Check sheet for the modelled part. Datum: model origin and axes. Units: mm. Face numbers are marked on the shaded views. Round coordinates to 2 decimals unless told otherwise and drop trailing zeros. Write each loop counter-clockwise with the first axis right and the second up, starting at its lowest first coordinate (ties: lowest second). Pieces come first, ordered by that corner, then holes. Notation, with made-up numbers: (9, 0) -> (13, 0) arc R22 ccw to (13, 32) -> close; hole circle Ø6 at (-16.5, -37). An arc over 180 degrees is marked (long way). Answer as a JSON object with one key per item and string values. Group by question number.
```python
from build123d import *

# Parameters (mm, degrees)
SKETCH_1_W               = 45
SKETCH_1_H               = 45
EXTRUDE_1_DEPTH          = 4
SKETCH_2_R               = 7.5
CUT_EXTRUDE_1_DEPTH      = 33.070235422
CUT_EXTRUDE_START        = -4.5
SKETCH_4_R               = 1.1
CUT_EXTRUDE_3_DEPTH      = 51.888424881
SKETCH_10_R              = 0.4
CUT_EXTRUDE_9_DEPTH      = 2
SKETCH_7_R               = 1.1
CUT_EXTRUDE_5_DEPTH      = 52.18645266
SKETCH_11_R              = 0.4
CUT_EXTRUDE_10_DEPTH     = 2
CUT_EXTRUDE_4_DEPTH      = 2
PATTERN_CIRCULAR_1_COUNT = 2
SKETCH_6_R               = 1.5
CUT_EXTRUDE_6_DEPTH      = 33.070235434
SKETCH_8_R               = 4.25
CUT_EXTRUDE_7_DEPTH      = 33.070235434
SKETCH_9_R               = 6
CUT_EXTRUDE_8_DEPTH      = 1
SKETCH_12_R              = 1.4
CUT_EXTRUDE_11_DEPTH     = 33.070235434
CHAMFER_1_SIZE           = 1
CHAMFER_2_SIZE           = 1
CHAMFER_3_SIZE           = 2


with BuildPart() as part:
    # 草图1 → 凸台-拉伸1 (new body)
    with BuildSketch(Plane(origin=(0, 0, 0), x_dir=(1, 0, 0), z_dir=(0, 1, 0))):
        Rectangle(SKETCH_1_W, SKETCH_1_H)
    extrude(amount=EXTRUDE_1_DEPTH)

    # 草图2 → 切除-拉伸1 (cut, through all)
    with BuildSketch(Plane(origin=(0, 4, 0), x_dir=(1, 0, 0), z_dir=(0, 1, 0))):
        with Locations(Location((0, 3, 0), (0, 0, 270))):
            Circle(SKETCH_2_R)
    extrude(amount=-CUT_EXTRUDE_1_DEPTH, mode=Mode.SUBTRACT)

    # 草图4 → 切除-拉伸3 (cut)
    with BuildSketch(Plane(origin=(-11.782001231, 4, -8.494037403), x_dir=(-0.4226182617407036, 0, 0.9063077870366482), z_dir=(-0.9063077870366482, 0, -0.4226182617407036)).offset(CUT_EXTRUDE_START)):
        Circle(SKETCH_4_R)
    cut_extrude_3 = extrude(amount=CUT_EXTRUDE_3_DEPTH, mode=Mode.SUBTRACT)

    # 草图10 → 切除-拉伸9 (cut)
    with BuildSketch(Plane(origin=(-8.852682854, 0, -4.12807381), x_dir=(-0.4226182617407035, 0, 0.906307787036648), z_dir=(-0.906307787036648, 0, -0.4226182617407035))):
        with Locations((-2.718923361, 4)):
            Circle(SKETCH_10_R)
    cut_extrude_9 = extrude(amount=-CUT_EXTRUDE_9_DEPTH, mode=Mode.SUBTRACT)

    # 草图7 → 切除-拉伸5 (cut)
    with BuildSketch(Plane(origin=(11.258330249, 4, -9.5), x_dir=(-0.5000000000000042, 0, -0.8660254037844363), z_dir=(0.8660254037844363, 0, -0.5000000000000042)).offset(CUT_EXTRUDE_START)):
        Circle(SKETCH_7_R)
    cut_extrude_5 = extrude(amount=CUT_EXTRUDE_5_DEPTH, mode=Mode.SUBTRACT)

    # 草图11 → 切除-拉伸10 (cut)
    with BuildSketch(Plane(origin=(8.660254038, 0, -5), x_dir=(-0.5000000000000042, 0, -0.8660254037844363), z_dir=(0.8660254037844363, 0, -0.5000000000000042))):
        with Locations((2.598076211, 4)):
            Circle(SKETCH_11_R)
    cut_extrude_10 = extrude(amount=-CUT_EXTRUDE_10_DEPTH, mode=Mode.SUBTRACT)

    # 草图5 → 切除-拉伸4 (cut)
    with BuildSketch(Plane(origin=(0, 4, 0), x_dir=(1, 0, 0), z_dir=(0, 1, 0))):
        Polygon((-11.782001231, 8.494037403), (-12.246881319, 7.497098837), (-12.415928624, 7.134575722), (-21.479006494, 11.360758339), (-20.211151709, 14.079681701), (-11.148073839, 9.853499083), (-11.317121144, 9.490975968), align=None)
        Polygon((12.008330249, 8.200961894), (10.508330249, 10.799038106), (19.168584287, 15.799038106), (20.668584287, 13.200961894), align=None)
    cut_extrude_4 = extrude(amount=-CUT_EXTRUDE_4_DEPTH, mode=Mode.SUBTRACT)

    # 阵列(圆周)1: 切除-拉伸3, 切除-拉伸9, 切除-拉伸5, 切除-拉伸10, 切除-拉伸4 ×2 about axis
    pattern_circular_1_axis = Axis((0, 0, -3), (0, 1, 0))
    add([cut_extrude_3.rotate(pattern_circular_1_axis, i * 360 / PATTERN_CIRCULAR_1_COUNT) for i in range(1, PATTERN_CIRCULAR_1_COUNT)], mode=Mode.SUBTRACT)
    add([cut_extrude_9.rotate(pattern_circular_1_axis, i * 360 / PATTERN_CIRCULAR_1_COUNT) for i in range(1, PATTERN_CIRCULAR_1_COUNT)], mode=Mode.SUBTRACT)
    add([cut_extrude_5.rotate(pattern_circular_1_axis, i * 360 / PATTERN_CIRCULAR_1_COUNT) for i in range(1, PATTERN_CIRCULAR_1_COUNT)], mode=Mode.SUBTRACT)
    add([cut_extrude_10.rotate(pattern_circular_1_axis, i * 360 / PATTERN_CIRCULAR_1_COUNT) for i in range(1, PATTERN_CIRCULAR_1_COUNT)], mode=Mode.SUBTRACT)
    add([cut_extrude_4.rotate(pattern_circular_1_axis, i * 360 / PATTERN_CIRCULAR_1_COUNT) for i in range(1, PATTERN_CIRCULAR_1_COUNT)], mode=Mode.SUBTRACT)

    # 草图6 → 切除-拉伸6 (cut, through all)
    with BuildSketch(Plane.XZ):
        with Locations(Location((19.5, -19.5, 0), (0, 0, 270))):
            Circle(SKETCH_6_R)
        with Locations(Location((-19.5, -19.5, 0), (0, 0, 270))):
            Circle(SKETCH_6_R)
        with Locations(Location((-19.5, 19.5, 0), (0, 0, 270))):
            Circle(SKETCH_6_R)
        with Locations(Location((19.5, 19.5, 0), (0, 0, 270))):
            Circle(SKETCH_6_R)
    extrude(amount=-CUT_EXTRUDE_6_DEPTH, mode=Mode.SUBTRACT)

    # 草图8 → 切除-拉伸7 (cut, through all)
    with BuildSketch(Plane(origin=(0, 4, 0), x_dir=(1, 0, 0), z_dir=(0, 1, 0))):
        with Locations(Location((0, -14.5, 0), (0, 0, 270))):
            Circle(SKETCH_8_R)
    extrude(amount=-CUT_EXTRUDE_7_DEPTH, mode=Mode.SUBTRACT)

    # 草图9 → 切除-拉伸8 (cut)
    with BuildSketch(Plane.XZ):
        with Locations(Location((0, 14.5, 0), (0, 0, 270))):
            Circle(SKETCH_9_R)
    extrude(amount=-CUT_EXTRUDE_8_DEPTH, mode=Mode.SUBTRACT)

    # 草图12 → 切除-拉伸11 (cut, through all)
    with BuildSketch(Plane(origin=(0, 0, 0), x_dir=(1, 0, 0), z_dir=(0, 1, 0))):
        with Locations(Location((0, 17.5, 0), (0, 0, 90))):
            Circle(SKETCH_12_R)
        with Locations(Location((-12, -15.5, 0), (0, 0, 90))):
            Circle(SKETCH_12_R)
        with Locations(Location((12, -15.5, 0), (0, 0, 90))):
            Circle(SKETCH_12_R)
    extrude(amount=CUT_EXTRUDE_11_DEPTH, mode=Mode.SUBTRACT)

    # 倒角1
    chamfer_1_edges = [part.edges().sort_by_distance(p)[0] for p in [
        (0, 1, 20.5),
    ]]
    chamfer(chamfer_1_edges, length=CHAMFER_1_SIZE - 0.0001)  # a hair under: the kernel refuses the full size

    # 倒角2
    chamfer_2_edges = [part.edges().sort_by_distance(p)[0] for p in [
        (22.5, 2, 22.5),
        (-22.5, 2, 22.5),
        (-22.5, 2, -22.5),
        (22.5, 2, -22.5),
    ]]
    chamfer(chamfer_2_edges, length=CHAMFER_2_SIZE)

    # 倒角3
    chamfer_3_edges = [part.edges().sort_by_distance(p)[0] for p in [
        (0, 0, -16.1),
        (-12, 0, 16.9),
        (12, 0, 16.9),
    ]]
    chamfer(chamfer_3_edges, length=CHAMFER_3_SIZE)


solid = part.part
```
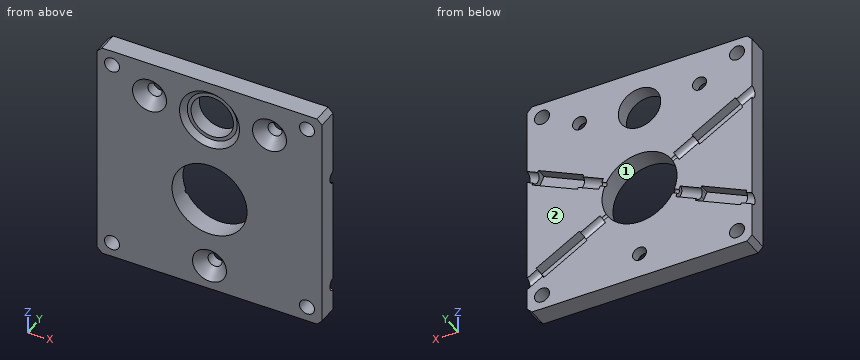
(1) Section check A-A on x = 0. State how many separate pieces and enclosed holes the cut face has, then the cut area to 3 significant figures.
(2) Scan lines: line 1 along X through (y, z) = (3, 19.5); line 2 along X through (y, z) = (1.1, 16.5); line 3 along X through (y, z) = (2.45, 14.5). Record each from-to range of solid material in increasing order.
(3) Release check for a two-part mould opening along X. For the marked faces 1 and 2 record: pulls with the +X half, pulls with the -X half, needs draft (parallel to the pull), parting line crosses it, or undercut.
(4) Section check B-B on z = -3. Record the cut outline in (x, y).
(5) Go/stop test with flat-tipped pins: pin 1 Ø5 at (x, z) = (0.5, 16.5) entering from -Y; pin 2 Ø3.5 at (x, z) = (0, -17.5) entering from -Y; pin 3 Ø4.5 at (x, z) = (12, 15.5) entering from -Y. Record where each tip stops, or that it passes through.
Data:
{
 "1": {"separate pieces": "4", "enclosed holes": "0", "area": "68.3 mm²"},
 "2": {"line 1": "x = -22.5 to -21, -18 to 18, 21 to 22.5", "line 2": "x = -22.5 to -14.07, -9.93 to -3.75, 3.75 to 9.93, 14.07 to 22.5", "line 3": "x = -22.5 to -12.98, -11.02 to -4.25, 4.25 to 11.02, 12.98 to 22.5"},
 "3": {"face 1": "undercut", "face 2": "needs draft"},
 "4": {"outline": "(-22.5, 0) -> (-7.5, 0) -> (-7.5, 4) -> (-22.5, 4) -> close; (7.5, 0) -> (22.5, 0) -> (22.5, 4) -> (7.5, 4) -> close"},
 "5": {"pin 1": "stops at y = 1", "pin 2": "stops at y = 1.65", "pin 3": "stops at y = 1.15"}
}
